Answer from the drawing. Dimensions are ordinates in mm from the lowest x, y and z of the part. A direction names the side the tool comes from. Coordinates: 2 decimals unless noted, no trailing zeros. Order: outer loops, then holes, each group sorted by start corner. A loop starts at its lowest first (then second) coordinate and runs counter-clockwise, first axis right, second up. Notation, with made-up numbers: (-39.5, 10) -> (8.5, 10) arc R25 cw to (8.5, 38) -> close; hole circle Ø2 at (-22.5, 80.25). An arc over 180 degrees is marked (long way). Answer in a Markdown table with one row per item.
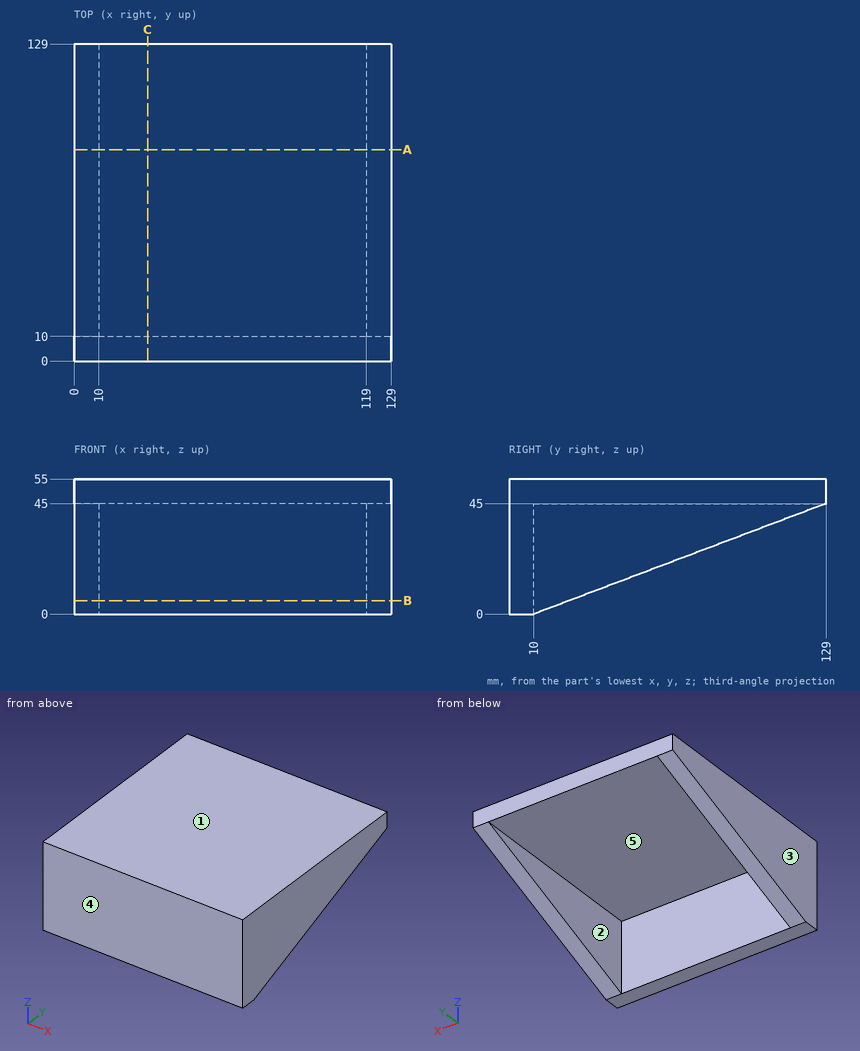
(1) For a pull along X with two mould halves and no side action, classify the marked faces 1, 2 and 3 as released by +X, released by -X, zero draft, split by the parting line, or undercut.
Check values:
| item | result |
|---|---|
| face 1 | zero draft |
| face 2 | undercut |
| face 3 | released by -X |
(2) A cutting plane is placed at C-C, the plane x = 30. Determine the outline of the cut face in (y, z), then the cut area to 3 significant figures.
Check values:
| item | result |
|---|---|
| outline | (0, 0) -> (10, 0) -> (10, 45) -> (129, 45) -> (129, 55) -> (0, 55) -> close |
| area | 1,740 mm² |
(3) A cutting plane is placed at B-B, the plane z = 5.5. Determine the outline of the cut face in (x, y), then the cut area to 3 significant figures.
Check values:
| item | result |
|---|---|
| outline | (0, 0) -> (129, 0) -> (129, 24.54) -> (119, 24.54) -> (119, 10) -> (10, 10) -> (10, 24.54) -> (0, 24.54) -> close |
| area | 1,580 mm² |
(4) Which of the six approach directions +Z, -Z, +X, -X, +Y, -Y give full straight-line access (tool end or side, diameter ignored) to the marked faces 4 and 5?
Check values:
| item | result |
|---|---|
| face 4 | +Z, -Z, +X, -X, -Y |
| face 5 | -Z, +Y |
(5) Flat-ended cylindrical pins translate along their axes: pin 1 (22.5 mm diameter, centred on x = 47, z = 22, fed in from +Y); pin 2 (1.5 mm diameter, centred on x = 110.5, y = 88, fed in from -Z). Find the tip coordinate at first contact, or state that the pin passes through.
Check values:
| item | result |
|---|---|
| pin 1 | y = 10 |
| pin 2 | z = 45 |
(6) Find the intervals of material crossed by line 1 along X through (y, z) = (54.5, 22); line 2 along Y through (x, z) = (47.5, 14); line 3 along Z through (x, y) = (48, 111.5), in increasing order. Write a range as from..to.
Check values:
| item | result |
|---|---|
| line 1 | 0..10, 119..129 |
| line 2 | 0..10 |
| line 3 | 45..55 |
(7) A cutting plane is placed at A-A, the plane y = 86. Determine the outline of the cut face in (x, z), then the cut area to 3 significant figures.
Check values:
| item | result |
|---|---|
| outline | (0, 28.74) -> (10, 28.74) -> (10, 45) -> (119, 45) -> (119, 28.74) -> (129, 28.74) -> (129, 55) -> (0, 55) -> close |
| area | 1,620 mm² |
